The figure shows three views and two pictorial views of one solid part (mm, origin at its lowest corner). Answer the questions. Round coordinates to 2 decimals unless told otherwise and drop trailing zeros. Write each loop counter-clockwise with the first axis right and the second up, starting at its lowest first coordinate (ties: lowest second). Pieces come first, ordered by that corner, then holes. Notation, with made-up numbers: (82, -16.5) - (99, -16.5) arc R17 ccw to (99, -7.5) - close; hole circle Ø8 at (13.5, -23.75). An arc over 180 degrees is marked (long way). Answer as CSV lines item,"result". Start each with the question number.
Item 1: A cutting plane is placed at B-B on z = 39. Determine the outline of the cut face in (x, y).
Item 2: A cutting plane is placed at A-A on y = 2.95. Determine the outline of the cut face in (x, z).
Item 3: A cutting plane is placed at C-C on x = 174.5. Determine the outline of the cut face in (y, z).
Item 4: Straight lines are drawn through the part: line 1 along X through (y, z) = (1.95, 47); line 2 along X through (y, z) = (2.8, 19); line 3 along Z through (x, y) = (137.5, 4.55). For each, find the intervals that lie inside material, in ascending order. Write a range as [from, to].
Item 5: Flat-ended cylindrical pins translate along their axes: pin 1 (1.5 mm diameter, centred on x = 6.5, y = 1.5, fed in from +Z); pin 2 (2 mm diameter, centred on y = 3, z = 32, fed in from -X); pin 3 (1.5 mm diameter, centred on y = 2, z = 64, fed in from -X); pin 4 (2.5 mm diameter, centred on y = 2, z = 13, fed in from +X). Find the tip coordinate at first contact, or state that the pin passes through.
Item 6: A cutting plane is placed at D-D on z = 15. Determine the outline of the cut face in (x, y), and give its area (3 significant figures).
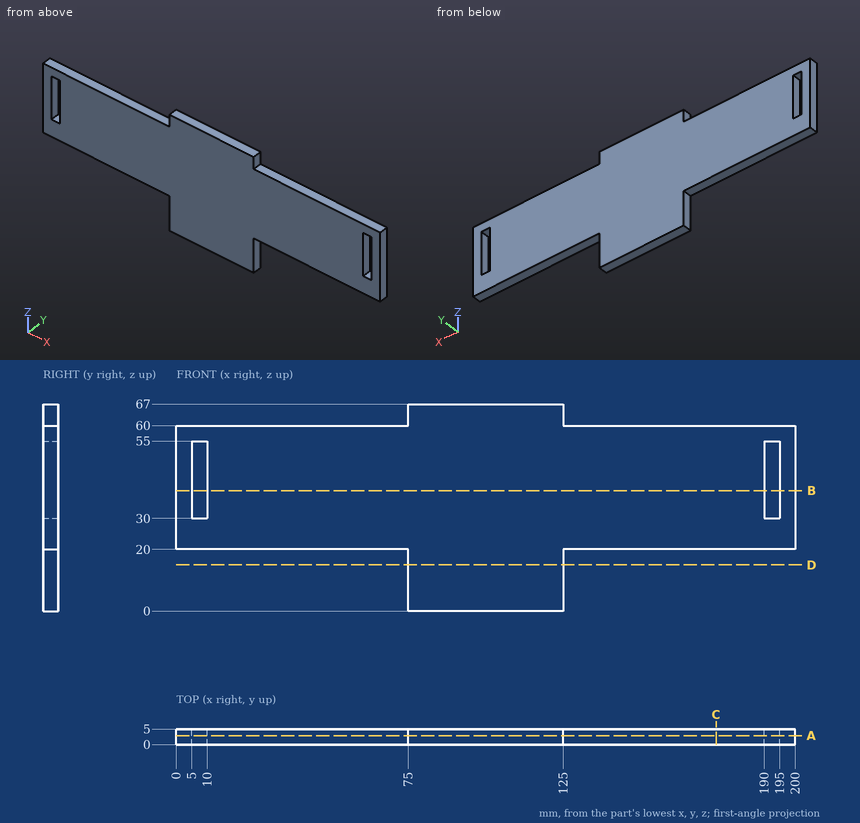
Geometry says:
1,outline,"(0, 0) - (5, 0) - (5, 5) - (0, 5) - close; (10, 0) - (190, 0) - (190, 5) - (10, 5) - close; (195, 0) - (200, 0) - (200, 5) - (195, 5) - close"
2,outline,"(0, 20) - (75, 20) - (75, 0) - (125, 0) - (125, 20) - (200, 20) - (200, 60) - (125, 60) - (125, 67) - (75, 67) - (75, 60) - (0, 60) - close; hole (5, 30) - (10, 30) - (10, 55) - (5, 55) - close; hole (190, 30) - (195, 30) - (195, 55) - (190, 55) - close"
3,outline,"(0, 20) - (5, 20) - (5, 60) - (0, 60) - close"
4,line 1,"x = [0, 5], [10, 190], [195, 200]"
4,line 2,"x = [75, 125]"
4,line 3,"z = [20, 60]"
5,pin 1,"stops at z = 60"
5,pin 2,"stops at x = 0"
5,pin 3,"stops at x = 75"
5,pin 4,"stops at x = 125"
6,outline,"(75, 0) - (125, 0) - (125, 5) - (75, 5) - close"
6,area,"250 mm^2"
